```python
from build123d import *

# Parameters (mm, degrees)
ESQUISSE1_W             = 40.6
ESQUISSE1_H             = 50
BOSS_EXTRU_1_DEPTH      = 8
ESQUISSE2_W             = 12
ESQUISSE2_H             = 50
BOSS_EXTRU_2_DEPTH      = 42.44
CHANFREIN1_SIZE         = 18
ESQUISSE3_R             = 24
BOSS_EXTRU_3_DEPTH      = 3
ESQUISSE4_R             = 14
BOSS_EXTRU_4_DEPTH      = 9
ESQUISSE5_W             = 20
ESQUISSE5_H             = 8
BOSS_EXTRU_5_DEPTH      = 8
CHANFREIN2_SIZE         = 5
CHANFREIN3_SIZE         = 5
ESQUISSE6_R             = 5.5
ENL_V_MAT_EXTRU_1_DEPTH = 81.244733381
ESQUISSE7_R             = 5.5
ENL_V_MAT_EXTRU_2_DEPTH = 80.655939168
ESQUISSE8_R             = 2
ENL_V_MAT_EXTRU_3_DEPTH = 81.244733381


with BuildPart() as part:
    # Esquisse1 → Boss.-Extru.1 (new body)
    with BuildSketch(Plane(origin=(0, 0, 0), x_dir=(1, 0, 0), z_dir=(0, 1, 0))):
        with Locations((-26.686076334, 4.522111117)):
            Rectangle(ESQUISSE1_W, ESQUISSE1_H)
    extrude(amount=BOSS_EXTRU_1_DEPTH)

    # Esquisse2 → Boss.-Extru.2 (add)
    with BuildSketch(Plane(origin=(0, 0, 0), x_dir=(-1, 0, 0), z_dir=(0, -1, 0))):
        with Locations((12.386076334, 4.522111117)):
            Rectangle(ESQUISSE2_W, ESQUISSE2_H)
    extrude(amount=BOSS_EXTRU_2_DEPTH)

    # Chanfrein1
    chanfrein1_edges = [part.edges().sort_by_distance(p)[0] for p in [
        (-12.386076334, -42.44, 20.477888883),
    ]]
    chamfer(chanfrein1_edges, length=CHANFREIN1_SIZE)

    # Esquisse3 → Boss.-Extru.3 (add)
    with BuildSketch(Plane(origin=(-6.386076334, 0, 0), x_dir=(0, 0, -1), z_dir=(1, 0, 0))):
        with Locations(Location((4.522111117, -17.44, 0), (0, 0, 205.528779366))):
            Circle(ESQUISSE3_R)
    extrude(amount=BOSS_EXTRU_3_DEPTH)

    # Esquisse4 → Boss.-Extru.4 (add)
    with BuildSketch(Plane(origin=(-3.386076334, 0, 0), x_dir=(0, 0, -1), z_dir=(1, 0, 0))):
        with Locations((4.522111117, -17.44)):
            Circle(ESQUISSE4_R)
    extrude(amount=BOSS_EXTRU_4_DEPTH)

    # Esquisse5 → Boss.-Extru.5 (add)
    with BuildSketch(Plane.ZY.offset(46.986076334)):
        with Locations((-4.522111117, 4)):
            Rectangle(ESQUISSE5_W, ESQUISSE5_H)
    extrude(amount=BOSS_EXTRU_5_DEPTH)

    # Chanfrein2
    chanfrein2_edges = [part.edges().sort_by_distance(p)[0] for p in [
        (-54.986076334, 4, 5.477888883),
    ]]
    chamfer(chanfrein2_edges, length=CHANFREIN2_SIZE)

    # Chanfrein3
    chanfrein3_edges = [part.edges().sort_by_distance(p)[0] for p in [
        (-54.986076334, 4, -14.522111117),
    ]]
    chamfer(chanfrein3_edges, length=CHANFREIN3_SIZE)

    # Esquisse6 → Enlèv. mat.-Extru.1 (cut, through all)
    with BuildSketch(Plane(origin=(0, 8, 0), x_dir=(1, 0, 0), z_dir=(0, 1, 0))):
        with Locations(Location((-37.986076334, 4.522111117, 0), (0, 0, 270))):
            Circle(ESQUISSE6_R)
    extrude(amount=-ENL_V_MAT_EXTRU_1_DEPTH, mode=Mode.SUBTRACT)

    # Esquisse7 → Enlèv. mat.-Extru.2 (cut, through all)
    with BuildSketch(Plane(origin=(5.613923666, 0, 0), x_dir=(0, 0, -1), z_dir=(1, 0, 0))):
        with Locations((4.522111117, -17.44)):
            Circle(ESQUISSE7_R)
    extrude(amount=-ENL_V_MAT_EXTRU_2_DEPTH, mode=Mode.SUBTRACT)

    # Esquisse8 → Enlèv. mat.-Extru.3 (cut, through all)
    with BuildSketch(Plane(origin=(0, 8, 0), x_dir=(1, 0, 0), z_dir=(0, 1, 0))):
        with Locations(Location((-41.486076334, -14.977888883, 0), (0, 0, 270))):
            Circle(ESQUISSE8_R)
        with Locations(Location((-41.486076334, 24.022111117, 0), (0, 0, 270))):
            Circle(ESQUISSE8_R)
    extrude(amount=-ENL_V_MAT_EXTRU_3_DEPTH, mode=Mode.SUBTRACT)


solid = part.part
```
Design review of the part built by this model. Coordinates are the model's own, in mm. A direction names the side the tool comes from. Coordinates: 2 decimals unless noted, no trailing zeros. Order: outer loops, then holes, each group sorted by start corner. A loop starts at its lowest first (then second) coordinate and runs counter-clockwise, first axis right, second up. Notation, with made-up numbers: (-23, -22.75) - (20, -22.75) arc R18 cw to (20, -13.75) - close; hole circle Ø5 at (-38, 11). An arc over 180 degrees is marked (long way). One line per question, with ' | ' between items.
Q1. Consider section D-D, the plane y = 3. Give the boundary of the cut face in (x, z), then the cut area to 3 significant figures.
Answer key:
outline: (-54.99, -9.52) - (-49.99, -14.52) - (-46.99, -14.52) - (-46.99, -29.52) - (-6.39, -29.52) - (-6.39, -17.1) - (-3.39, -17.1) - (-3.39, 8.06) - (-6.39, 8.06) - (-6.39, 20.48) - (-46.99, 20.48) - (-46.99, 5.48) - (-49.99, 5.48) - (-54.99, 0.48) - close; hole circle Ø4 at (-41.49, -24.02); hole circle Ø11 at (-37.99, -4.52); hole circle Ø4 at (-41.49, 14.98) | area: 2,120 mm2
Q2. Consider section B-B, the plane x = -36.5. Give the boundary of the cut face in (y, z).
Answer key:
outline: (0, -29.52) - (8, -29.52) - (8, -9.82) - (0, -9.82) - close; (0, 0.77) - (8, 0.77) - (8, 20.48) - (0, 20.48) - close
Q3. To check wall thickness, follow line 1 along Y through (x, z) = (-27, -8); line 2 along X through (y, z) = (-10, 13.5); line 3 along Z through (x, y) = (-8, -17). State the ranges of each line that lie inside material, in increasing order.
Answer key:
line 1: y = 0 to 8 | line 2: x = -18.39 to -3.39 | line 3: z = -29.52 to -10, 0.96 to 20.48
Q4. Consider section C-C, the plane z = -20.5. Give the boundary of the cut face in (x, y), then the cut area to 3 significant figures.
Answer key:
outline: (-46.99, 0) - (-18.39, 0) - (-18.39, -42.44) - (-6.39, -42.44) - (-6.39, -35.35) - (-3.39, -35.35) - (-3.39, 0.47) - (-6.39, 0.47) - (-6.39, 8) - (-46.99, 8) - close | area: 942 mm2
Q5. Clearance check with flat-ended pins moving along their axes: pin 1 Ø2.5 at (y, z) = (5.5, 11.5) entering from -X; pin 2 Ø2 at (y, z) = (-3, 13) entering from +X; pin 3 Ø4 at (y, z) = (-14.5, -7) entering from +X; pin 4 Ø3 at (x, z) = (-43, -2) entering from -Y. State where each tip first meets the part, or that it passes through.
Answer key:
pin 1: stops at x = -46.99 | pin 2: stops at x = -3.39 | pin 3: stops at x = 5.61 | pin 4: stops at y = 0
Q6. Consider section A-A, the plane y = -17.44. Give the boundary of the cut face in (x, z), then the cut area to 3 significant figures.
Answer key:
outline: (-18.39, -29.52) - (-6.39, -29.52) - (-6.39, -28.52) - (-3.39, -28.52) - (-3.39, -18.52) - (5.61, -18.52) - (5.61, -10.02) - (-18.39, -10.02) - close; (-18.39, 0.98) - (5.61, 0.98) - (5.61, 9.48) - (-3.39, 9.48) - (-3.39, 19.48) - (-6.39, 19.48) - (-6.39, 20.48) - (-18.39, 20.48) - close | area: 732 mm2
Q7. The part is to be moulded in two halves that separate along Z. For faces 6 (the cylindrical face through (-39.8, 4.06, -22.95)), 7 (the flat face through (-52.521, 3.944, 2.943)), 8 (the flat face through (-46.986, 4, -22)), say which applies: +Z half, -Z half, draft (parallel to the pull), parting line (faces both ways), or undercut.
Answer key:
face 6: undercut | face 7: +Z half | face 8: draft
Q8. For faces 1 (the flat face through (-29, 0, -5)), 2 (the flat face through (-12.3, -33.57, 11.35)), 3 (the flat face through (-54.986, 4, -5)), 4 (the flat face through (-46.986, 4, 13)), 5 (the flat face through (-3.386, -13, 9)), list the 3-axis set-ups (+Z, -Z, +X, -X, +Y, -Y) from which the entire face can be reached by the end or side of a thin tool; tool diameter is ignored.
Answer key:
face 1: +Z, -Z, -X, -Y | face 2: +Z, -X, -Y | face 3: +Z, -Z, -X, +Y, -Y | face 4: +Z, -X, +Y, -Y | face 5: +X
